Autodesk Inventor part; units mm, degrees
ref_plane "YZ Plane" through (0, 0, 0) normal (1, 0, 0) x (0, 1, 0)
ref_plane "XZ Plane" through (0, 0, 0) normal (0, 1, 0) x (-1, 0, 0)
ref_plane "XY Plane" through (0, 0, 0) normal (0, 0, 1) x (1, 0, 0)
sketch "Sketch1" plane through (0, 0, 0) normal (1, 0, 0) x (0, 1, 0)
  line L0 (48, 50) -> (-48, 50)
  line L1 (-48, 50) -> (-48, -50)
  line L2 (-48, -50) -> (48, -50)
  line L3 (48, -50) -> (48, 50)
  point P0 (0, 0)
  dimension "d0" = 96
  dimension "d1" = 100
  dimension "d2" = 50
  dimension "d3" = 48
extrude "Extrusion1" add sketch "Sketch1" along normal blind 1.5
sketch "Sketch2" plane through (0, -48, 50) normal (0, 0, 1) x (1, 0, 0)
  line L0 (0, 96) -> (1.5, 96)
  line L1 (1.5, 96) -> (-7, 96)
  line L2 (-7, 96) -> (-7, 0)
  line L3 (-7, 0) -> (1.5, 0)
  line L4 (1.5, 0) -> (1.5, 96)
  point P0 (0, 48)
  dimension "d6" = 8.5
  dimension "d7" = 96
extrude "Extrusion2" add sketch "Sketch2" against normal blind 1.5
mirror "Mirror1" about plane through (0, 0, 0) normal (0, 0, 1) of "Extrusion2"
fillet "Fillet1" radius 0.5 2 edges at (1.5, 0, 50) (1.5, 0, -50)
sketch "Sketch12" plane through (-7, -48, 48.5) normal (0, -1, 0) x (1, 0, 0)
  arc A0 (8, -98.5) -> (8.5, -98) centre (8, -98) ccw
  line L0 (8.5, 1) -> (8.5, -98)
  arc A1 (8.5, 1) -> (8, 1.5) centre (8, 1) ccw
  line L1 (0, 1.5) -> (8, 1.5)
  line L2 (0, 1.5) -> (0, 0)
  line L3 (7, 0) -> (0, 0)
  line L4 (7, 0) -> (7, -97)
  line L5 (7, -97) -> (0, -97)
  line L6 (0, -98.5) -> (0, -97)
  line L7 (0, -98.5) -> (8, -98.5)
  point P0 (7, -48.5)
extrude "Extrusion8" add sketch "Sketch12" along normal blind 56.75
sketch "Sketch13" plane through (-7, 48, 48.5) normal (0, 1, 0) x (1, 0, 0)
  arc A0 (8.5, 98) -> (8, 98.5) centre (8, 98) ccw
  line L0 (0, 98.5) -> (8, 98.5)
  line L1 (0, 98.5) -> (0, 97)
  line L2 (0, 97) -> (7, 97)
  line L3 (7, 97) -> (7, 0)
  line L4 (0, 0) -> (7, 0)
  line L5 (0, -1.5) -> (0, 0)
  line L6 (8, -1.5) -> (0, -1.5)
  arc A1 (8, -1.5) -> (8.5, -1) centre (8, -1) ccw
  line L7 (8.5, 98) -> (8.5, -1)
  point P0 (7, 48.5)
extrude "Extrusion9" add sketch "Sketch13" along normal blind 56.75
sketch "Sketch14" plane through (1.5, 0, 0) normal (1, 0, 0) x (0, 0, -1)
  line L0 (49.5, -104.75) -> (49.5, 104.75)
  line L1 (-49.5, 104.75) -> (49.5, 104.75)
  line L2 (-49.5, 104.75) -> (-49.5, -104.75)
  line L3 (49.5, -104.75) -> (-49.5, -104.75)
  line L4 (0, 0) -> (-23.5475, 0) construction
  point P0 (35, -100.75)
  point P1 (-35, -100.75)
  point P2 (35, 100.75)
  point P3 (-35, 100.75)
  dimension "d88" = 70
  dimension "d89" = 35
  dimension "d90" = 4
hole "Hole6" at (1.5, -100.75, -35) at (1.5, -100.75, 35) at (1.5, 100.75, -35) at (1.5, 100.75, 35) direction (-1, 0, 0) diameter 3.454 end through all
sketch "Sketch15" plane through (1.5, 0, 0) normal (1, 0, 0) x (0, 0, -1)
  circle A0 centre (25, -48) radius 1.727
  circle A1 centre (-25, -48) radius 1.727
  circle A2 centre (25, 48) radius 1.727
  circle A3 centre (-25, 48) radius 1.727
  point P0 (0, 0)
hole "Hole7" at (1.5, -48, -25) at (1.5, -48, 25) at (1.5, 48, -25) at (1.5, 48, 25) direction (-1, 0, 0) diameter 3.454 end through all
sketch "Sketch16" plane through (0, 0, 0) normal (-1, 0, 0) x (0, 0, 1)
  line L0 (38.5, 69.75) -> (48.5, 69.75)
  line L1 (48.5, 69.75) -> (48.5, 84.75)
  line L2 (48.5, 84.75) -> (38.5, 84.75)
  line L3 (38.5, 84.75) -> (38.5, 69.75)
  circle A0 centre (-25, 48) radius 1.727
  circle A1 centre (-25, -48) radius 1.727
  circle A2 centre (25, -48) radius 1.727
  circle A3 centre (25, 48) radius 1.727
  circle A4 centre (-35, 100.75) radius 1.727
  circle A5 centre (-35, -100.75) radius 1.727
  circle A6 centre (35, -100.75) radius 1.727
  circle A7 centre (35, 100.75) radius 1.727
  line L4 (-48.5, 104.75) -> (-48.5, -104.75)
  line L5 (48.5, -104.75) -> (-48.5, -104.75)
  line L6 (48.5, -104.75) -> (48.5, 104.75)
  line L7 (-48.5, 104.75) -> (48.5, 104.75)
  line L8 (48.5, -104.75) -> (48.5, 104.75)
  point P0 (0, 0)
  dimension "d105" = 10
  dimension "d106" = 15
  dimension "d107" = 20
extrude "Extrusion10" add sketch "Sketch16" along normal blind 0.8 contours L3 L2 L1 L0
sketch "Sketch17" plane through (-0.8, 0, 0) normal (-1, 0, 0) x (0, 0, 1)
  line L0 (38.5, 69.75) -> (48.5, 69.75)
  line L1 (48.5, 84.75) -> (48.5, 69.75)
  line L2 (48.5, 84.75) -> (38.5, 84.75)
  line L3 (38.5, 84.75) -> (38.5, 69.75)
  line L4 (38.5, 69.75) -> (48.5, 69.75)
  point P0 (0, 0)
  point P1 (42.9, 75.25)
  point P2 (42.9, 79.25)
  dimension "d110" = 4
  dimension "d111" = 5.5
  dimension "d123" = 5.6
hole "Hole8" at (-0.8, 75.25, 42.9) at (-0.8, 79.25, 42.9) direction (1, 0, 0) diameter 1.1811 depth 1.651
mirror "Mirror2" about plane through (0, 0, 0) normal (0, 0, 1) of "Extrusion10", "Hole8"
sketch "Sketch18" plane through (0, -48, 48.5) normal (0, 0, -1) x (-1, 0, 0)
  line L0 (0.8, 132.75) -> (0.8, 117.75)
  line L1 (0, 132.75) -> (0.8, 132.75)
  line L2 (0.8, 132.75) -> (3.8, 132.75)
  line L3 (3.8, 132.75) -> (3.8, 117.75)
  line L4 (3.8, 117.75) -> (0.8, 117.75)
  line L5 (0.8, 117.75) -> (0.8, 132.75)
  point P0 (0, 48)
  dimension "d119" = 3
  dimension "d120" = 15
extrude "Extrusion11" cut sketch "Sketch18" against normal through all
mirror "Mirror3" about plane through (0, 0, 0) normal (0, 0, 1) of "Extrusion11"
chamfer "Chamfer1" distance 2 angle 45 4 edges at (-0.4, 69.75, -38.5) (-0.4, 84.75, -38.5) (-0.4, 69.75, 38.5) (-0.4, 84.75, 38.5)
properties part number "memesat shear panel type 1" material "Aluminum 6061"
Geometry check sheet. Reference: the model listing, model coordinates, mm. Give positions to 0.01 mm unless a question says otherwise; leave off trailing zeros. Order: outer loops, then holes, each group sorted by start corner. A loop starts at its lowest first (then second) coordinate and runs counter-clockwise, first axis right, second up. Notation, with made-up numbers: (-9.5, 52.5) - (14.5, 52.5) arc R17 cw to (14.5, 63.5) - close; hole circle Ø8 at (85.5, -17.75). An arc over 180 degrees is marked (long way). Use one line per item in the form item = value.
1) Sectioned sample at B-B (y = -36.5). Record the boundary of the cut face in (x, z).
Working result:
outline = (-7, -50) - (1, -50) arc R0.5 ccw to (1.5, -49.5) - (1.5, 49.5) arc R0.5 ccw to (1, 50) - (-7, 50) - (-7, 48.5) - (0, 48.5) - (0, -48.5) - (-7, -48.5) - close
2) Sectioned sample at C-C (z = -20). Record the boundary of the cut face in (x, y), and give its area (3 significant figures).
Working result:
outline = (0, -104.75) - (1.5, -104.75) - (1.5, 104.75) - (0, 104.75) - close
area = 314 mm^2
3) Material ranges on probe 1 along Y at (x, z) = (0.55, -25); probe 2 along Z at (x, y) = (-0.35, 79.25); probe 3 along Z at (x, y) = (1, 100.75), recorded low to high. Write a range as from..to.
Working result:
probe_1 = -104.75..-49.73, -46.27..46.27, 49.73..104.75
probe_2 = -50..-43.49, -42.31..-38.5, 38.5..42.31, 43.49..50
probe_3 = -50..-36.73, -33.27..33.27, 36.73..50
4) Depth check by flat-ended pin: pin 1 Ø1.3 at (y, z) = (75, -42.5) entering from -X; pin 2 Ø3 at (y, z) = (49.5, -9) entering from -X. Enter the tip coordinate at first touch or a pass-through.
Working result:
pin_1 = -0.8
pin_2 = 0
5) Sectioned sample at A-A (x = -5.5). Record the boundary of the cut face in (y, z).
Working result:
outline = (-104.75, -50) - (104.75, -50) - (104.75, -48.5) - (-104.75, -48.5) - close; (-104.75, 48.5) - (104.75, 48.5) - (104.75, 50) - (-104.75, 50) - close
